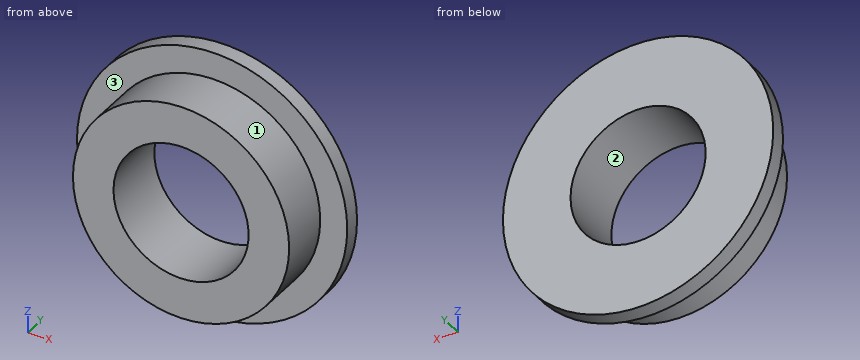
Autodesk Inventor part; units mm, degrees
ref_plane "YZ Plane" through (0, 0, 0) normal (1, 0, 0) x (0, 1, 0)
ref_plane "XZ Plane" through (0, 0, 0) normal (0, 1, 0) x (-1, 0, 0)
ref_plane "XY Plane" through (0, 0, 0) normal (0, 0, 1) x (1, 0, 0)
sketch "スケッチ1" plane through (0, 0, 0) normal (0, 1, 0) x (-1, 0, 0)
  circle A0 centre (0, 0) radius 4
  circle A1 centre (0, 0) radius 2.5
  dimension "d0" = 8
  dimension "d1" = 5
extrude "押し出し1" add sketch "スケッチ1" along normal blind 2
sketch "スケッチ2" plane through (0, 2, 0) normal (0, 1, 0) x (1, 0, 0)
  circle A0 centre (0, 0) radius 5
  dimension "d4" = 10
extrude "押し出し2" add sketch "スケッチ2" along normal blind 1
sketch "スケッチ3" plane through (0, 3, 0) normal (0, 1, 0) x (1, 0, 0)
  circle A0 centre (0, 0) radius 5
extrude "押し出し3" cut sketch "スケッチ3" against normal blind 0.4
sketch "スケッチ4" plane through (0, 2.6, 0) normal (0, 1, 0) x (1, 0, 0)
  circle A0 centre (0, 0) radius 2.5
  circle A1 centre (0, 0) radius 2.5
  dimension "d9" = 5
extrude "押し出し4" cut sketch "スケッチ4" against normal blind 0.6
sketch "スケッチ5" plane through (0, 0, 0) normal (0, -1, 0) x (1, 0, 0)
  circle A0 centre (0, 0) radius 2.5
  circle A1 centre (0, 0) radius 4
extrude "押し出し5" cut sketch "スケッチ5" against normal blind 0.1
properties part number "SMF85 ベアリング" material "ステンレス鋼"
Part model, mm, in its own coordinate system. Face numbers are marked on the shaded views. Coordinates: 2 decimals unless noted, no trailing zeros. Loops run counter-clockwise (first coordinate to the right, second up) from the corner with the lowest first, then second, coordinate; pieces in that order, holes last. Notation, with made-up numbers: (13, 0) - (24, 0) arc R22 cw to (24, 16) - close; hole circle Ø9 at (-17.75, 49). An arc over 180 degrees is marked (long way). Write item = value, one per line. Start each with the question number.
Item 1: Flat gauge pins, fed straight in: pin 1 Ø3 at (x, z) = (0, 0) entering from +Y; pin 2 Ø1 at (x, y) = (-2, 0.5) entering from -Z. Where does each tip first touch, or does it go through?
Item 2: Cut at A-A, the plane z = 0. Give the cut face in (x, y).
Item 3: Cut at C-C, the plane x = 3.25. Give the cut face in (y, z), and give its area (3 significant figures).
Item 4: Wall check: L1, parallel to Z at x = 0, y = 1.35; L2, parallel to Z at x = -0.75, y = 1.8; L3, parallel to X at y = 2.4, z = 2.25. Give the ranges that are in metal, low to high. Write a range as from..to.
Item 5: Cut at D-D, the plane y = 1.25. Give the cut face in (x, z).
Item 6: Cut at B-B, the plane x = 0. Give the cut face in (y, z), and give its area (3 significant figures).
Item 7: Mould opens along Z. For the marked faces 1, 2 and 3 say: released by +Z, released by -Z, zero draft, split by the parting line, or undercut.
The answers:
q1.pin_1 = through
q1.pin_2 = -3.71
q2.outline = (-5, 2) - (-4, 2) - (-4, 0.1) - (-2.5, 0.1) - (-2.5, 2.6) - (-5, 2.6) - close; (2.5, 0.1) - (4, 0.1) - (4, 2) - (5, 2) - (5, 2.6) - (2.5, 2.6) - close
q3.outline = (0.1, -2.33) - (2, -2.33) - (2, -3.8) - (2.6, -3.8) - (2.6, 3.8) - (2, 3.8) - (2, 2.33) - (0.1, 2.33) - close
q3.area = 13.4 mm2
q4.L1 = -4..-2.5, 2.5..4
q4.L2 = -3.93..-2.38, 2.38..3.93
q4.L3 = -4.47..-1.09, 1.09..4.47
q5.outline = circle Ø8 at (0, 0); hole circle Ø5 at (0, 0)
q6.outline = (0.1, -4) - (2, -4) - (2, -5) - (2.6, -5) - (2.6, -2.5) - (0.1, -2.5) - close; (0.1, 2.5) - (2.6, 2.5) - (2.6, 5) - (2, 5) - (2, 4) - (0.1, 4) - close
q6.area = 8.70 mm2
q7.face_1 = split by the parting line
q7.face_2 = undercut
q7.face_3 = zero draft
